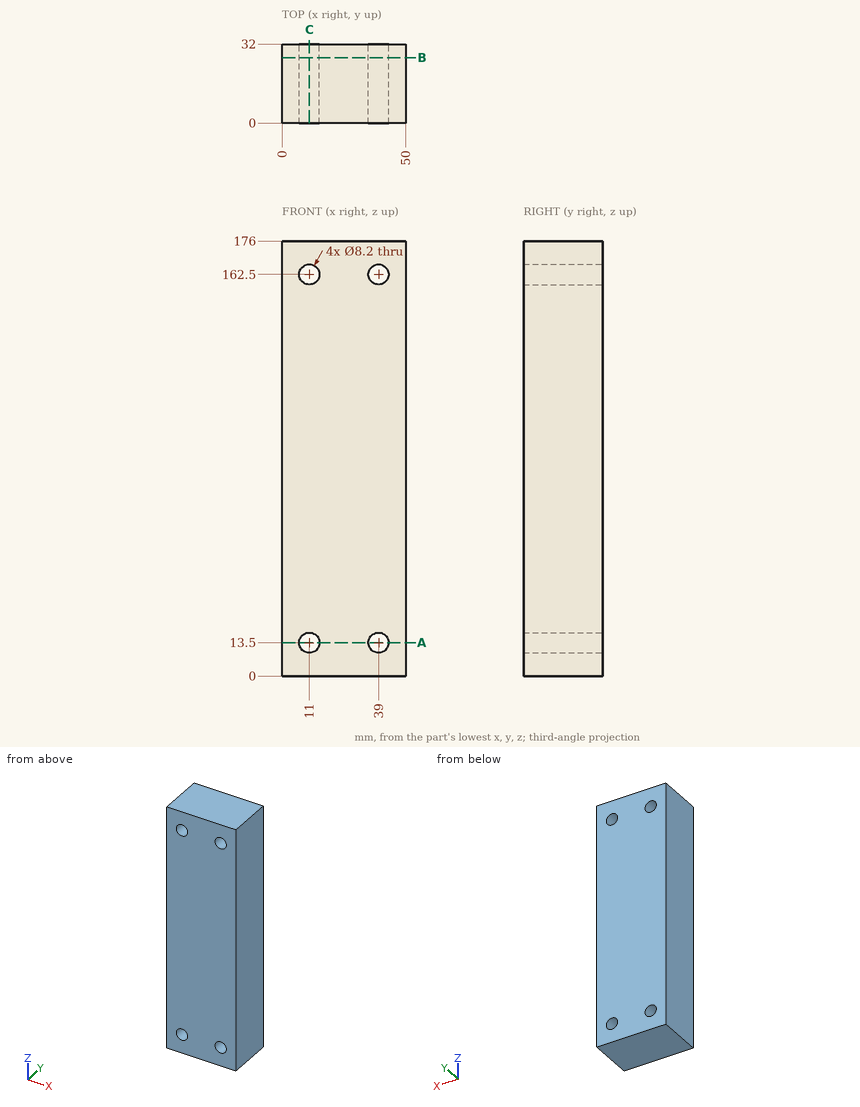
Verification items for this drawing (mm, ordinates from the low corner). Give positions to 0.01 mm unless a question says otherwise; leave off trailing zeros. Loops run counter-clockwise (first coordinate to the right, second up) from the corner with the lowest first, then second, coordinate; pieces in that order, holes last. Notation, with made-up numbers: (1.5, -23) - (55.5, -23) arc R17 ccw to (55.5, 0) - close; hole circle Ø6 at (80.5, -8). An arc over 180 degrees is marked (long way). Write item = value, one per line. Start each with the question number.
Q1. Thickness scan on line 1 (X direction, y = 9, z = 162); line 2 (Z direction, x = 11, y = 24); line 3 (Z direction, x = 9, y = 11.5). Record the ranges inside material, lowest first.
Q2. Cross-section at B-B, the plane y = 26.5. Enter the section's corners in (x, z).
Q3. Depth check by flat-ended pin: P1, Ø10.5, axis at x = 11, z = 162.5, coming from the -Y side. Enter the tip coordinate at first touch or a pass-through.
Q4. Cross-section at C-C, the plane x = 11. Enter the section's corners in (y, z), and give its area (3 significant figures).
Q5. Cross-section at A-A, the plane z = 13.5. Enter the section's corners in (x, y).
Answer key:
q1.line_1 = 0 to 6.93, 15.07 to 34.93, 43.07 to 50
q1.line_2 = 0 to 9.4, 17.6 to 158.4, 166.6 to 176
q1.line_3 = 0 to 9.92, 17.08 to 158.92, 166.08 to 176
q2.outline = (0, 0) - (50, 0) - (50, 176) - (0, 176) - close; hole circle Ø8.2 at (11, 13.5); hole circle Ø8.2 at (11, 162.5); hole circle Ø8.2 at (39, 13.5); hole circle Ø8.2 at (39, 162.5)
q3.P1 = 0
q4.outline = (0, 0) - (32, 0) - (32, 9.4) - (0, 9.4) - close; (0, 17.6) - (32, 17.6) - (32, 158.4) - (0, 158.4) - close; (0, 166.6) - (32, 166.6) - (32, 176) - (0, 176) - close
q4.area = 5,110 mm^2
q5.outline = (0, 0) - (6.9, 0) - (6.9, 32) - (0, 32) - close; (15.1, 0) - (34.9, 0) - (34.9, 32) - (15.1, 32) - close; (43.1, 0) - (50, 0) - (50, 32) - (43.1, 32) - close
